Verification items for the finished model (mm, model axes). Face numbers are marked on the shaded views. Give positions to 0.01 mm unless a question says otherwise; leave off trailing zeros. Loops run counter-clockwise (first coordinate to the right, second up) from the corner with the lowest first, then second, coordinate; pieces in that order, holes last. Notation, with made-up numbers: (50.5, 34) - (70.5, 34) arc R28 ccw to (70.5, 61) - close; hole circle Ø2 at (-18, -27). An arc over 180 degrees is marked (long way). Answer in a Markdown table with one row per item.
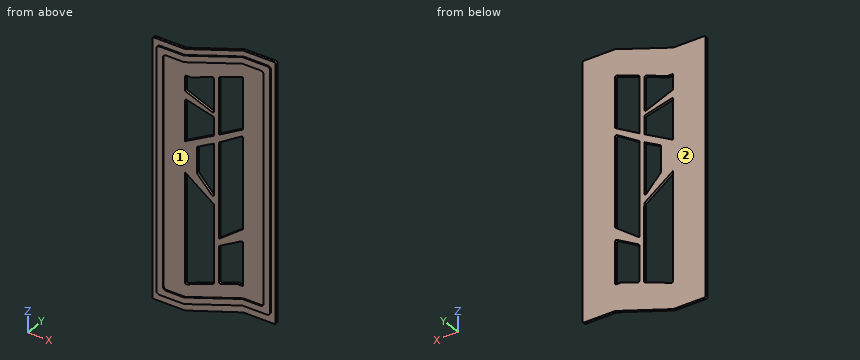
```python
from build123d import *

# Parameters (mm, degrees)
F1_DEPTH = 4
F3_DEPTH = 6


with BuildPart() as f1:
    # F0 (on Front) → F1 (new body)
    with BuildSketch(Plane.XZ):
        with BuildLine():
            ThreePointArc((0.311493, 77.652204), (-0.004355, 77.573432), (-0.328798, 77.54694))
            Line((-0.328798, 77.54694), (-48, 77.54694))
            ThreePointArc((-48, 77.54694), (-49.414214, 76.961154), (-50, 75.54694))
            Line((-50, 75.54694), (-50, -320.45306))
            ThreePointArc((-50, -320.45306), (-49.414214, -321.867273), (-48, -322.45306))
            Line((-48, -322.45306), (-0.324555, -322.45306))
            ThreePointArc((-0.324555, -322.45306), (-0.004191, -322.427235), (0.3079, -322.350426))
            Line((0.3079, -322.350426), (89.6921, -292.555693))
            ThreePointArc((89.6921, -292.555693), (90.004191, -292.478885), (90.324555, -292.45306))
            Line((90.324555, -292.45306), (138, -292.45306))
            ThreePointArc((138, -292.45306), (139.414214, -291.867273), (140, -290.45306))
            Line((140, -290.45306), (140, 105.960753))
            ThreePointArc((140, 105.960753), (139.414214, 107.374967), (138, 107.960753))
            Line((138, 107.960753), (90.328798, 107.960753))
            ThreePointArc((90.328798, 107.960753), (90.004355, 107.934262), (89.688507, 107.85549))
            Line((89.688507, 107.85549), (0.311493, 77.652204))
        make_face()
        with BuildLine():
            ThreePointArc((0.08659, 34.963099), (0.392042, 36.736965), (1.999475, 37.54694))
            Line((1.999475, 37.54694), (9.632653, 37.54694))
            ThreePointArc((9.632653, 37.54694), (9.993956, 37.579846), (10.34337, 37.67748))
            Line((10.34337, 37.67748), (41.702027, 50.270872))
            ThreePointArc((41.702027, 50.270872), (43.567476, 50.071842), (44.447355, 48.414939))
            Line((44.447355, 48.414939), (44.531555, 2.188108))
            Line((44.531555, 2.188108), (44.538406, -1.573441))
            Line((44.538406, -1.573441), (44.55651, -11.512594))
            Line((44.55651, -11.512594), (44.567509, -17.551468))
            Line((44.567509, -17.551468), (44.603887, -37.523114))
            Line((44.603887, -37.523114), (44.603911, -37.536671))
            Line((44.603911, -37.536671), (44.606063, -38.717808))
            Line((44.606063, -38.717808), (44.628078, -50.804465))
            Line((44.628078, -50.804465), (44.634246, -54.191019))
            Line((44.634246, -54.191019), (44.771094, -129.322448))
            Line((44.771094, -129.322448), (44.799309, -144.812723))
            Line((44.799309, -144.812723), (44.806541, -148.783601))
            Line((44.806541, -148.783601), (44.892246, -195.836749))
            Line((44.892246, -195.836749), (44.951897, -228.585603))
            Line((44.951897, -228.585603), (44.952764, -229.062129))
            Line((44.952764, -229.062129), (44.956313, -231.010533))
            Line((44.956313, -231.010533), (44.957229, -231.513005))
            Line((44.957229, -231.513005), (45.015878, -263.712596))
            ThreePointArc((45.015878, -263.712596), (44.666439, -264.84569), (43.736825, -265.581779))
            Line((43.736825, -265.581779), (2.702247, -281.439717))
            ThreePointArc((2.702247, -281.439717), (1.115069, -281.36063), (0.08659, -280.149176))
            Line((0.08659, -280.149176), (0.08659, -213.666722))
            Line((0.08659, -213.666722), (0.08659, -213.666518))
            Line((0.08659, -213.666518), (0.08659, -109.831086))
            Line((0.08659, -109.831086), (0.08659, -64.548373))
            Line((0.08659, -64.548373), (0.08659, -3.747635))
            Line((0.08659, -3.747635), (0.08659, -1.128253))
            Line((0.08659, -1.128253), (0.08659, 14.797802))
            Line((0.08659, 14.797802), (0.08659, 18.424725))
            Line((0.08659, 18.424725), (0.08659, 34.963099))
        make_face(mode=Mode.SUBTRACT)
        with BuildLine():
            ThreePointArc((90, -250.45306), (89.414214, -251.867273), (88, -252.45306))
            Line((88, -252.45306), (80.362669, -252.45306))
            ThreePointArc((80.362669, -252.45306), (80.00582, -252.485153), (79.660422, -252.580401))
            Line((79.660422, -252.580401), (55.136718, -261.70943))
            ThreePointArc((55.136718, -261.70943), (53.302525, -261.471919), (52.447355, -259.831991))
            Line((52.447355, -259.831991), (52.447355, -208.675399))
            Line((52.447355, -208.675399), (52.447355, -205.710266))
            Line((52.447355, -205.710266), (52.447355, -192.655353))
            Line((52.447355, -192.655353), (52.447355, -191.636056))
            Line((52.447355, -191.636056), (52.447355, -46.193009))
            Line((52.447355, -46.193009), (52.447355, -34.354303))
            Line((52.447355, -34.354303), (52.447355, 52.370707))
            ThreePointArc((52.447355, 52.370707), (52.799274, 53.503769), (53.731183, 54.238084))
            Line((53.731183, 54.238084), (87.289282, 66.930212))
            ThreePointArc((87.289282, 66.930212), (89.135466, 66.707178), (90, 65.060752))
            Line((90, 65.060752), (90, -10.053347))
            Line((90, -10.053347), (90, -11.364244))
            Line((90, -11.364244), (90, -26.140187))
            Line((90, -26.140187), (90, -29.092925))
            Line((90, -29.092925), (90, -158.712357))
            Line((90, -158.712357), (90, -163.930135))
            Line((90, -163.930135), (90, -186.452676))
            Line((90, -186.452676), (90, -189.093262))
            Line((90, -189.093262), (90, -250.45306))
        make_face(mode=Mode.SUBTRACT)
        with BuildLine():
            ThreePointArc((86.933276, -24.448412), (88.966062, -24.38898), (90, -26.140187))
            Line((90, -26.140187), (90, -11.364244))
            ThreePointArc((90, -11.364244), (89.733629, -12.361506), (89.005469, -13.093126))
            Line((89.005469, -13.093126), (52.447355, -34.354303))
            Line((52.447355, -34.354303), (52.447355, -46.193009))
            Line((52.447355, -46.193009), (86.933276, -24.448412))
        make_face()
        with BuildLine():
            ThreePointArc((1.336144, 12.943933), (0.428143, 13.679967), (0.08659, 14.797802))
            Line((0.08659, 14.797802), (0.08659, -1.128253))
            ThreePointArc((0.08659, -1.128253), (0.860722, 0.452015), (2.583838, 0.808947))
            Line((2.583838, 0.808947), (43.053761, -9.579037))
            ThreePointArc((43.053761, -9.579037), (44.135664, -10.288931), (44.55651, -11.512594))
            Line((44.55651, -11.512594), (44.538406, -1.573441))
            ThreePointArc((44.538406, -1.573441), (43.657754, -3.234512), (41.787964, -3.430953))
            Line((41.787964, -3.430953), (1.336144, 12.943933))
        make_face()
        with BuildLine():
            ThreePointArc((1.117742, -62.798706), (0.363555, -63.532917), (0.08659, -64.548373))
            Line((0.08659, -64.548373), (0.08659, -109.831086))
            ThreePointArc((0.08659, -109.831086), (0.30142, -110.732846), (0.89976, -111.44088))
            Line((0.89976, -111.44088), (43.986142, -143.206573))
            ThreePointArc((43.986142, -143.206573), (44.583659, -143.912981), (44.799309, -144.812723))
            Line((44.799309, -144.812723), (44.771094, -129.322448))
            ThreePointArc((44.771094, -129.322448), (43.498808, -131.189002), (41.298194, -130.679071))
            Line((41.298194, -130.679071), (19.18674, -106.607738))
            ThreePointArc((19.18674, -106.607738), (18.796071, -105.980772), (18.659644, -105.254758))
            Line((18.659644, -105.254758), (18.659644, -66.362716))
            ThreePointArc((18.659644, -66.362716), (18.936609, -65.347259), (19.690796, -64.613049))
            Line((19.690796, -64.613049), (44.628078, -50.804465))
            Line((44.628078, -50.804465), (44.606063, -38.717808))
            Line((44.606063, -38.717808), (1.117742, -62.798706))
        make_face()
        with BuildLine():
            ThreePointArc((87.004425, -184.718078), (89.00221, -184.721903), (90, -186.452676))
            Line((90, -186.452676), (90, -163.930135))
            ThreePointArc((90, -163.930135), (89.792549, -164.817134), (89.213233, -165.520124))
            Line((89.213233, -165.520124), (53.189984, -193.007491))
            ThreePointArc((53.189984, -193.007491), (52.707297, -193.066297), (52.447355, -192.655353))
            Line((52.447355, -192.655353), (52.447355, -205.710266))
            ThreePointArc((52.447355, -205.710266), (52.716582, -204.708056), (53.45178, -203.975668))
            Line((53.45178, -203.975668), (87.004425, -184.718078))
        make_face()
    extrude(amount=F1_DEPTH)

    # F2 (on face) → F3 (join)
    with BuildSketch(Plane.XZ):
        with BuildLine():
            Line((132.914576, -275.868222), (132.914576, 94.131778))
            ThreePointArc((132.914576, 94.131778), (131.45011, 97.667312), (127.914576, 99.131778))
            Line((127.914576, 99.131778), (90.743754, 99.131778))
            ThreePointArc((90.743754, 99.131778), (89.925748, 99.064411), (89.129784, 98.864124))
            Line((89.129784, 98.864124), (0.784792, 68.733994))
            ThreePointArc((0.784792, 68.733994), (-0.011172, 68.533708), (-0.829178, 68.46634))
            Line((-0.829178, 68.46634), (-38, 68.46634))
            ThreePointArc((-38, 68.46634), (-41.535534, 67.001874), (-43, 63.46634))
            Line((-43, 63.46634), (-43, -306.53366))
            ThreePointArc((-43, -306.53366), (-41.535534, -310.069194), (-38, -311.53366))
            Line((-38, -311.53366), (-0.829178, -311.53366))
            ThreePointArc((-0.829178, -311.53366), (-0.011172, -311.466292), (0.784792, -311.266006))
            Line((0.784792, -311.266006), (89.129784, -281.135876))
            ThreePointArc((89.129784, -281.135876), (89.925748, -280.935589), (90.743754, -280.868222))
            Line((90.743754, -280.868222), (127.914576, -280.868222))
            ThreePointArc((127.914576, -280.868222), (131.45011, -279.403756), (132.914576, -275.868222))
        make_face()
        with BuildLine():
            ThreePointArc((122.914576, -265.868222), (121.45011, -269.403756), (117.914576, -270.868222))
            Line((117.914576, -270.868222), (90.743754, -270.868222))
            ThreePointArc((90.743754, -270.868222), (89.925748, -270.935589), (89.129784, -271.135876))
            Line((89.129784, -271.135876), (0.784792, -301.266006))
            ThreePointArc((0.784792, -301.266006), (-0.011172, -301.466292), (-0.829178, -301.53366))
            Line((-0.829178, -301.53366), (-28, -301.53366))
            ThreePointArc((-28, -301.53366), (-31.535534, -300.069194), (-33, -296.53366))
            Line((-33, -296.53366), (-33, 53.46634))
            ThreePointArc((-33, 53.46634), (-31.535534, 57.001874), (-28, 58.46634))
            Line((-28, 58.46634), (-0.829178, 58.46634))
            ThreePointArc((-0.829178, 58.46634), (-0.011172, 58.533708), (0.784792, 58.733994))
            Line((0.784792, 58.733994), (89.129784, 88.864124))
            ThreePointArc((89.129784, 88.864124), (89.925748, 89.064411), (90.743754, 89.131778))
            Line((90.743754, 89.131778), (117.914576, 89.131778))
            ThreePointArc((117.914576, 89.131778), (121.45011, 87.667312), (122.914576, 84.131778))
            Line((122.914576, 84.131778), (122.914576, -265.868222))
        make_face(mode=Mode.SUBTRACT)
    extrude(amount=F3_DEPTH)


solid = f1.part
```
Q1. Sectioned sample at B-B (x = -18). Record the cut outline in (y, z), and give its area (3 significant figures).
Completed:
| item | result |
|---|---|
| outline | (-6, -311.53) - (-4, -311.53) - (-4, -322.45) - (0, -322.45) - (0, 77.55) - (-4, 77.55) - (-4, 68.47) - (-6, 68.47) - (-6, 58.47) - (-4, 58.47) - (-4, -301.53) - (-6, -301.53) - close |
| area | 1,640 mm^2 |
Q2. Sectioned sample at A-A (x = 75.5). Record the cut outline in (y, z).
Completed:
| item | result |
|---|---|
| outline | (-6, -285.78) - (-4, -285.78) - (-4, -297.29) - (0, -297.29) - (0, -254.13) - (-4, -254.13) - (-4, -275.78) - (-6, -275.78) - close; (-6, 84.22) - (-4, 84.22) - (-4, 62.47) - (0, 62.47) - (0, 103.06) - (-4, 103.06) - (-4, 94.22) - (-6, 94.22) - close; (-4, -191.32) - (0, -191.32) - (0, -175.98) - (-4, -175.98) - close; (-4, -31.66) - (0, -31.66) - (0, -20.95) - (-4, -20.95) - close |
Q3. Sectioned sample at C-C (y = -2). Give the number of separate pieces and of enclosed holes in the cut face, and give its area (3 significant figures).
Completed:
| item | result |
|---|---|
| separate pieces | 1 |
| enclosed holes | 7 |
| area | 53,100 mm^2 |
Q4. Draft check along X on the marked faces 1 and 2. Enter one of: +X half, -X half, draft (parallel to the pull), parting line (faces both ways), or undercut.
Completed:
| item | result |
|---|---|
| face 1 | undercut |
| face 2 | draft |
Q5. Thickness scan on line 1 (X direction, y = -1.1, z = -240.5); line 2 (X direction, y = -3.1, z = 33.5); line 3 (X direction, y = -5.5, z = -121). Record the ranges inside material, lowest first.
Completed:
| item | result |
|---|---|
| line 1 | -50 to 0.09, 44.97 to 52.45, 90 to 140 |
| line 2 | -50 to 0.09, 44.47 to 52.45, 90 to 140 |
| line 3 | -43 to -33, 122.91 to 132.91 |
Q6. Sectioned sample at D-D (z = -124). Record the cut outline in (x, y), and give its area (3 significant figures).
Completed:
| item | result |
|---|---|
| outline | (-50, -4) - (-43, -4) - (-43, -6) - (-33, -6) - (-33, -4) - (0.09, -4) - (0.09, 0) - (-50, 0) - close; (17.93, -4) - (35.16, -4) - (35.16, 0) - (17.93, 0) - close; (44.76, -4) - (52.45, -4) - (52.45, 0) - (44.76, 0) - close; (90, -4) - (122.91, -4) - (122.91, -6) - (132.91, -6) - (132.91, -4) - (140, -4) - (140, 0) - (90, 0) - close |
| area | 540 mm^2 |
Q7. Go/stop test with flat-tipped pins: P1, Ø4, axis at x = -26, z = -266.5, coming from the -Y side; P2, Ø1.5, axis at x = 53, y = -2, coming from the -Z side; P3, Ø2, axis at x = 5.5, y = -1, coming from the -Z side. Record where each tip stops, or that it passes through.
Completed:
| item | result |
|---|---|
| P1 | y = -4 |
| P2 | z = -305.04 |
| P3 | z = -320.95 |
